Input: part model. Units: mm. Frame: model coordinates. A direction names the side the tool comes from. Round coordinates to 2 decimals unless told otherwise and drop trailing zeros. Write each loop counter-clockwise with the first axis right and the second up, starting at its lowest first coordinate (ties: lowest second). Pieces come first, ordered by that corner, then holes. Notation, with made-up numbers: (44.5, -26) -> (52.5, -26) arc R6 ccw to (52.5, -22) -> close; hole circle Ø8 at (30.5, 84.5). An arc over 180 degrees is marked (long way). Use CSV: the item, a comma, the result in double quotes.
Autodesk Fusion 360 part; units mm, degrees
sketch "Sketch1" plane through (0, 0, 0) normal (0, 0, 1) x (1, 0, 0)
  line L0 (60, 37.5) -> (-60, 37.5)
  line L1 (-60, 37.5) -> (-60, -37.5)
  line L2 (-60, -37.5) -> (60, -37.5)
  line L3 (60, -37.5) -> (60, 37.5)
  line L4 (60, 37.5) -> (-60, -37.5) construction
  line L5 (-60, 37.5) -> (60, -37.5) construction
  line L6 (45, 20) -> (-45, 20)
  line L7 (-45, 20) -> (-45, -20)
  line L8 (-45, -20) -> (45, -20)
  line L9 (45, -20) -> (45, 20)
  line L10 (45, 20) -> (-45, -20) construction
  line L11 (-45, 20) -> (45, -20) construction
  line L12 (-40, 15) -> (40, 15)
  line L13 (40, 15) -> (40, -15)
  line L14 (40, -15) -> (-40, -15)
  line L15 (-40, -15) -> (-40, 15)
  line L16 (-40, 15) -> (40, -15) construction
  line L17 (40, 15) -> (-40, -15) construction
  dimension "d1" = 120
  dimension "d2" = 75
  dimension "d3" = 90
  dimension "d4" = 40
  dimension "d5" = 80
  dimension "d6" = 30
extrude "Extrude1" add sketch "Sketch1" along normal blind 20 makes body 1 at (15, -31.6667, 0) makes body 2 at (-13.3333, -5, 0)
extrude "Extrude2" add sketch "Sketch1" along normal blind 5 contours L6 L7 L8 L9 bodies 1 2
Item 1: Line query: line 1 (Y direction, x = 8, z = 8.5); line 2 (X direction, y = 1, z = 13.5); line 3 (X direction, y = 16, z = 12). Output: solid intervals per line, ascending.
Worked answers:
line 1,"y = -37.5 to -20, -15 to 15, 20 to 37.5"
line 2,"x = -60 to -45, -40 to 40, 45 to 60"
line 3,"x = -60 to -45, 45 to 60"
Item 2: Section query A-A on z = 15.25. Return the cut outline in (x, y), plus the area to 3 significant figures.
Worked answers:
outline,"(-60, -37.5) -> (60, -37.5) -> (60, 37.5) -> (-60, 37.5) -> close; (-40, -15) -> (40, -15) -> (40, 15) -> (-40, 15) -> close; hole (-45, -20) -> (45, -20) -> (45, 20) -> (-45, 20) -> close"
area,"7,800 mm²"
Item 3: Pull-direction query (Y, two-part tool) for faces 1 (the face through (-1, 26, 20)), 2 (the face through (-1, -20, 12)), 3 (the face through (-1, -37.5, 10)); classes: +Y half, -Y half, draft (parallel to the pull), parting line (faces both ways), or undercut.
Worked answers:
face 1,"draft"
face 2,"undercut"
face 3,"-Y half"
Item 4: Section query B-B on x = 26.5. Return the cut outline in (y, z), plus the area to 3 significant figures.
Worked answers:
outline,"(-37.5, 0) -> (37.5, 0) -> (37.5, 20) -> (20, 20) -> (20, 5) -> (15, 5) -> (15, 20) -> (-15, 20) -> (-15, 5) -> (-20, 5) -> (-20, 20) -> (-37.5, 20) -> close"
area,"1,350 mm²"
Item 5: Section query D-D on x = 43.5. Return the cut outline in (y, z).
Worked answers:
outline,"(-37.5, 0) -> (37.5, 0) -> (37.5, 20) -> (20, 20) -> (20, 5) -> (-20, 5) -> (-20, 20) -> (-37.5, 20) -> close"
Item 6: Section query C-C on y = -18. Return the cut outline in (x, z).
Worked answers:
outline,"(-60, 0) -> (60, 0) -> (60, 20) -> (45, 20) -> (45, 5) -> (-45, 5) -> (-45, 20) -> (-60, 20) -> close"
Item 7: Set-up query: faces 4 (the face through (1, 37.5, 10)), 5 (the face through (1, -15, 12)). Return all of +Z, -Z, +X, -X, +Y, -Y with unobstructed straight access to the full face (end or side cutting, diameter ignored); none if empty.
Worked answers:
face 4,"+Z, -Z, +X, -X, +Y"
face 5,"+Z"
